Autodesk Inventor part; units mm, degrees
ref_plane "YZ Plane" through (0, 0, 0) normal (1, 0, 0) x (0, 1, 0)
ref_plane "XZ Plane" through (0, 0, 0) normal (0, 1, 0) x (-1, 0, 0)
ref_plane "XY Plane" through (0, 0, 0) normal (0, 0, 1) x (1, 0, 0)
sketch "Эскиз1" plane through (0, 0, 0) normal (0, 1, 0) x (-1, 0, 0)
  circle A0 centre (16, 32.5) radius 1.75
  circle A1 centre (16, -17) radius 1.75
  circle A2 centre (-8, -17) radius 1.75
  circle A3 centre (-8, 32.5) radius 1.75
  line L0 (20.75, 37.25) -> (-12.75, 37.25)
  line L1 (-12.75, 37.25) -> (-12.75, -21.75)
  line L2 (-12.75, -21.75) -> (20.75, -21.75)
  line L3 (20.75, -21.75) -> (20.75, 37.25)
  point P0 (0, 0)
  dimension "d0" = 3.5
  dimension "d1" = 3.5
  dimension "d2" = 46
  dimension "d3" = 3.5
  dimension "d4" = 20.5
  dimension "d5" = 3.5
  dimension "d6" = 46
  dimension "d8" = 20.5
  dimension "d9" = 3
  dimension "d10" = 3
  dimension "d11" = 3
  dimension "d12" = 3
  dimension "d13" = 3
  dimension "d14" = 3
  dimension "d15" = 59
  dimension "d16" = 3
  dimension "d17" = 4.75
extrude "Выдавливание1" add sketch "Эскиз1" along normal blind 3
sketch "Эскиз2" plane through (0, 3, 0) normal (0, 1, 0) x (1, 0, 0)
  line L0 (-20.75, 21.75) -> (-20.75, -37.25)
  line L1 (-20.75, 3.25) -> (-17.75, 3.25)
  line L2 (-17.75, 3.25) -> (-17.75, -18.75)
  line L3 (-17.75, -18.75) -> (-20.75, -18.75)
  line L4 (-20.75, -18.75) -> (-20.75, 3.25)
  line L5 (12.75, -37.25) -> (12.75, 21.75)
  line L6 (12.75, 3.25) -> (9.75, 3.25)
  line L7 (9.75, 3.25) -> (9.75, -18.75)
  line L8 (9.75, -18.75) -> (12.75, -18.75)
  line L9 (12.75, -18.75) -> (12.75, 3.25)
  line L10 (12.75, 21.75) -> (-20.75, 21.75)
  line L11 (-20.75, -37.25) -> (12.75, -37.25)
  point P0 (0, 0)
  dimension "d20" = 59
  dimension "d21" = 3
  dimension "d22" = 3
  dimension "d23" = 22
  dimension "d24" = 22
  dimension "d25" = 18.5
  dimension "d26" = 18.5
  dimension "d27" = 18.5
extrude "Выдавливание2" add sketch "Эскиз2" along normal blind 30 contours L1 L2 L3 L0 | L5 L8 L7 L6
sketch "Эскиз3" plane through (0, 33, 0) normal (0, 1, 0) x (1, 0, 0)
  line L0 (-20.75, 21.75) -> (-20.75, 3.25)
  line L1 (-20.75, 24.75) -> (67.25, 24.75)
  line L2 (67.25, 24.75) -> (67.25, -40.25)
  line L3 (67.25, -40.25) -> (-20.75, -40.25)
  line L4 (-20.75, -40.25) -> (-20.75, 24.75)
  line L5 (12.75, 21.75) -> (-20.75, 21.75)
  line L6 (-20.75, -37.25) -> (12.75, -37.25)
  line L7 (69.25, 26.75) -> (-22.75, 26.75)
  line L8 (-22.75, 26.75) -> (-22.75, -42.25)
  line L9 (-22.75, -42.25) -> (69.25, -42.25)
  line L10 (69.25, -42.25) -> (69.25, 26.75)
  point P0 (0, 0)
  dimension "d30" = 88
  dimension "d31" = 65
  dimension "d34" = 59
  dimension "d35" = 88
  dimension "d38" = 3
  dimension "d39" = 2
  dimension "d40" = 2
  dimension "d41" = 2
  dimension "d42" = 2
extrude "Выдавливание3" add sketch "Эскиз3" along normal blind 3 contours L4 L1 L2 L3 L0
sketch "Эскиз4" plane through (0, 36, 0) normal (0, 1, 0) x (1, 0, 0)
  line L0 (67.25, 24.75) -> (-20.75, 24.75)
  line L1 (67.25, 24.75) -> (-20.75, 24.75)
  line L2 (-20.75, 24.75) -> (-20.75, -40.25)
  line L3 (-20.75, -40.25) -> (67.25, -40.25)
  line L4 (67.25, -40.25) -> (67.25, 24.75)
  line L5 (69.25, 26.75) -> (-22.75, 26.75)
  line L6 (-22.75, 26.75) -> (-22.75, -42.25)
  line L7 (-22.75, -42.25) -> (69.25, -42.25)
  line L8 (69.25, -42.25) -> (69.25, 26.75)
  line L9 (33.25, 26.75) -> (23.25, 26.75)
  line L10 (23.25, 24.75) -> (33.25, 24.75)
  line L11 (67.25, -40.25) -> (-20.75, -40.25)
  line L12 (30, -42.25) -> (40, -42.25)
  line L13 (40, -40.25) -> (30, -40.25)
  line L14 (28.25, 24.75) -> (18.25, 24.75)
  line L15 (18.25, 24.75) -> (18.25, 26.75)
  line L16 (18.25, 26.75) -> (28.25, 26.75)
  line L17 (28.25, 26.75) -> (28.25, 24.75)
  line L18 (18.25, -40.25) -> (28.25, -40.25)
  line L19 (28.25, -40.25) -> (28.25, -42.25)
  line L20 (28.25, -42.25) -> (18.25, -42.25)
  line L21 (18.25, -42.25) -> (18.25, -40.25)
  point P0 (0, 0)
  dimension "d43" = 2
  dimension "d44" = 2
  dimension "d45" = 2
  dimension "d46" = 2
  dimension "d51" = 10
  dimension "d52" = 41
  dimension "d53" = 41
  dimension "d54" = 10
  dimension "d55" = 41
extrude "Выдавливание4" add sketch "Эскиз4" along normal blind 12 and the other way blind 3 contours L0 L17 L5 L8 L7 L19 L3 L4 | L0 L2 L3 L21 L7 L6 L5 L15
fillet "Сопряжение1" radius 2 3 edges at (9.75, 3, 7.75) (11.25, 3, 18.75) (11.25, 3, -3.25)
fillet "Сопряжение2" radius 2 3 edges at (-19.25, 3, -3.25) (-17.75, 3, 7.75) (-19.25, 3, 18.75)
fillet "Сопряжение3" radius 2 8 edges at (11.25, 33, 18.75) (12.75, 33, 7.75) (-17.75, 33, 7.75) (-19.25, 33, 18.75) (-20.75, 33, 7.75) (-19.25, 33, -3.25) (9.75, 33, 7.75) (11.25, 33, -3.25)
fillet "Сопряжение4" radius 3 4 edges at (-20.75, 1.5, 37.25) (12.75, 1.5, 37.25) (-20.75, 1.5, -21.75) (12.75, 1.5, -21.75)
properties part number "батарейки"
Geometry check sheet. Reference: the model listing, model coordinates, mm. A direction names the side the tool comes from. Give positions to 0.01 mm unless a question says otherwise; leave off trailing zeros. Write each loop counter-clockwise with the first axis right and the second up, starting at its lowest first coordinate (ties: lowest second). Pieces come first, ordered by that corner, then holes. Notation, with made-up numbers: M -37,-15.5 L 15,-15.5 A17 ccw 15,-8.5 Z; hole C 20.25,40.25 d5. An arc over 180 degrees is marked long. One line per question, with ' | ' between items.
1. Cross-section at D-D (x = -3). Enter the section's corners in (y, z).
Ans:
outline: M 0,-21.75 L 3,-21.75 L 3,37.25 L 0,37.25 Z; M 33,-26.75 L 48,-26.75 L 48,-24.75 L 36,-24.75 L 36,40.25 L 48,40.25 L 48,42.25 L 33,42.25 Z
2. Cross-section at C-C (z = 32.5). Enter the section's corners in (x, y).
Ans:
outline: M -22.75,33 L 69.25,33 L 69.25,48 L 67.25,48 L 67.25,36 L -20.75,36 L -20.75,48 L -22.75,48 Z; M -20.75,0 L -17.75,0 L -17.75,3 L -20.75,3 Z; M -14.25,0 L 6.25,0 L 6.25,3 L -14.25,3 Z; M 9.75,0 L 12.75,0 L 12.75,3 L 9.75,3 Z
3. Mould release check, pull along Y, two halves, no side actions. Record for faces 4 (the face through (-4, 3, 8)), 5 (the face through (28.25, 40, 41)), 6 (the face through (9.15, 3.57, 7.93)): released by +Y, released by -Y, zero draft, split by the parting line, or undercut.
Ans:
face 4: undercut | face 5: zero draft | face 6: undercut
4. Cross-section at A-A (z = 25). Enter the section's corners in (x, y).
Ans:
outline: M -22.75,33 L 69.25,33 L 69.25,48 L 67.25,48 L 67.25,36 L -20.75,36 L -20.75,48 L -22.75,48 Z; M -20.75,0 L 12.75,0 L 12.75,3 L -20.75,3 Z
5. Set-up check for faces 1 (the face through (-4, 1, 37.25)), 2 (the face through (11.201, 32.626, -4.085)), 3 (the face through (-19.3, 32.65, 19.62)): record each of +Z, -Z, +X, -X, +Y, -Y from which the full face is reachable in a straight line by a thin tool's end or side.
Ans:
face 1: +Z, +X, -X, -Y | face 2: -Z, +X, -X | face 3: +Z, +X, -X
6. Scan lines: line 1 along Z through (x, y) = (8, 1.65); line 2 along Z through (x, y) = (41, 39); line 3 along Y through (x, z) = (-8, 3). Record each from-to range of solid material in increasing order. Write a range as from..to.
Ans:
line 1: -21.75..-18.75, -15.25..30.75, 34.25..37.25 | line 2: -26.75..-24.75, 40.25..42.25 | line 3: 0..3, 33..36
7. Gauge pin test, flat ends, axial feed: pin 1 (4.5 mm diameter, centred on x = 8, z = -17, fed in from +Y); pin 2 (2.5 mm diameter, centred on x = -10.5, y = 2, fed in from -Z); pin 3 (4 mm diameter, centred on x = 50, z = 20, fed in from -Y); pin 4 (12 mm diameter, centred on y = 28, z = -17.5, fed in from +X). Record the tip position at first contact, or that the pin passes through.
Ans:
pin 1: y = 36 | pin 2: z = -21.75 | pin 3: y = 33 | pin 4: x = 69.25
8. Cross-section at B-B (y = 45.5). Enter the section's corners in (x, z), plus the area to 3 significant figures.
Ans:
outline: M -22.75,-26.75 L 18.25,-26.75 L 18.25,-24.75 L -20.75,-24.75 L -20.75,40.25 L 18.25,40.25 L 18.25,42.25 L -22.75,42.25 Z; M 28.25,-26.75 L 69.25,-26.75 L 69.25,42.25 L 28.25,42.25 L 28.25,40.25 L 67.25,40.25 L 67.25,-24.75 L 28.25,-24.75 Z | area: 588 mm2
